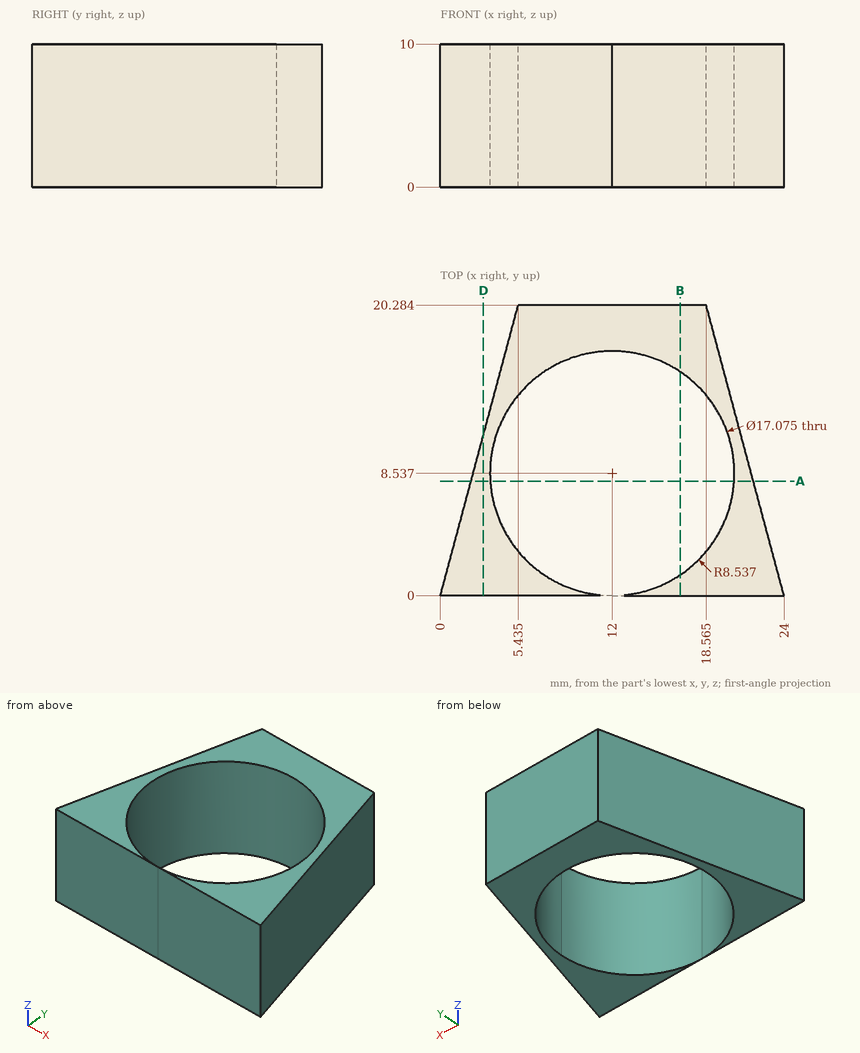
The figure shows three views and two pictorial views of one solid part (mm, origin at its lowest corner). Answer the questions. Round coordinates to 2 decimals unless told otherwise and drop trailing zeros. Order: outer loops, then holes, each group sorted by start corner. A loop starts at its lowest first (then second) coordinate and runs counter-clockwise, first axis right, second up. Notation, with made-up numbers: M 42,33.5 L 82,33.5 A18 ccw 82,67.5 Z; hole C -9.75,77.5 d9. An arc over 180 degrees is marked long. Answer in a Markdown table with one row per item. Add a question column.
1) The part is cut by section B-B on x = 16.75. Determine the outline of the cut face in (y, z) (1 decimal).
2) The part is cut by section D-D on x = 3. Determine the outline of the cut face in (y, z), plus the area to 3 significant figures.
3) Consider line 1 along X through (y, z) = (14.25, 4.5) (1 decimal); line 2 along Y through (x, z) = (17.25, 2.75) (1 decimal); line 3 along Y through (x, z) = (18.25, 2.25) (1 decimal). Determine where each line is inside the solid, lowest interval first. Write a range as from..to.
4) The part is cut by section A-A on y = 8. Determine the outline of the cut face in (x, z).
Findings below:
| question | item | result |
|---|---|---|
| 1 | outline | M 0,0 L 1.4,0 L 1.4,10 L 0,10 Z; M 15.6,0 L 20.3,0 L 20.3,10 L 15.6,10 Z |
| 2 | outline | M 0,0 L 11.2,0 L 11.2,10 L 0,10 Z |
| 2 | area | 112 mm² |
| 3 | line 1 | x = 3.8..5.7, 18.3..20.2 |
| 3 | line 2 | y = 0..1.8, 15.3..20.3 |
| 3 | line 3 | y = 0..2.7, 14.4..20.3 |
| 4 | outline | M 2.14,0 L 3.48,0 L 3.48,10 L 2.14,10 Z; M 20.52,0 L 21.86,0 L 21.86,10 L 20.52,10 Z |
